Solid Edge part; units mm, degrees
sketch "Sketch1" plane through (0, 0, 0) normal (0, -1, 0) x (1, 0, 0)
  line L0 (0, 0) -> (9, 0)
  line L1 (9, 0) -> (7.5, 3)
  line L2 (7.5, 3) -> (0, 3)
  dimension "D1" = 9
  dimension "D2" = 7.5
revolve "RevolvedProtrusion1" add sketch "Sketch1" angle 360 about axis through (0, 0, 3) along (0, 0, -1)
sketch "Sketch2" plane through (0, 0, 3) normal (0, 0, 1) x (1, 0, 0)
  line L0 (0, 4.6188) -> (-4, -2.3094)
  line L1 (-4, -2.3094) -> (4, -2.3094)
  line L2 (4, -2.3094) -> (0, 4.6188)
  dimension "D1" = 4
extrude "triangle_cut" cut sketch "Sketch2" against normal blind 0.5
fillet "Round1" radius 0.25 5 edges at (-9, 0, 0) (-7.5, 0, 3) (-2, 1.1547, 3) (2, 1.1547, 3) (0, -2.3094, 3)
properties material "Polyethylene, low density"
Here's how the part is built. I have some questions about the finished solid (model axes, mm). A direction names the side the tool comes from. Coordinates: 2 decimals unless noted, no trailing zeros. Order: outer loops, then holes, each group sorted by start corner. A loop starts at its lowest first (then second) coordinate and runs counter-clockwise, first axis right, second up. Notation, with made-up numbers: M -33.5,89 L 24.5,89 A22 ccw 24.5,105 Z; hole C 81,-1.5 d3. An arc over 180 degrees is marked long. Answer as a JSON object with one key per item and string values. Group by question number.
(1) Which directions (+Z, -Z, +X, -X, +Y, -Y) give clear straight access to the entire face, cutting with the end or side of a thin tool? Please do faces 5 (the face through (2.03, 1.24, 2.92)), 6 (the face through (0, 0, 0)).
(2) Suppose I cut it at A-A, the plane z = 1.95. Please give me the cut outline in (x, y) (3 decimals), then the cut area to 3 significant figures.
(3) If we mould it in two halves opening along Y, with no side actions, what happens to faces 1 (the face through (3.2, -0.1, 3)), 2 (the face through (-2.093, 1.137, 2.925)), 3 (the face through (0, 0, 2.5)), 4 (the face through (7.29, -2.3, 2.71))? For each: released by +Y, released by -Y, zero draft, split by the parting line, or undercut.
(4) Suppose I cut it at B-B, the plane z = 0.85. Please give me the cut outline in (x, y) (3 decimals), then the cut area to 3 significant figures.
(5) I need wall thicknesses on probe 1 along Y at (x, z) = (1.75, 2.55); probe 2 along X at (y, z) = (-2.25, 2.65); probe 3 along X at (y, z) = (0, 0.4). Which ranges of each line are inside material? Lowest first, please.
Values found:
{
 "1": {"face 5": "+Z", "face 6": "-Z, +X, -X, +Y, -Y"},
 "2": {"outline": "C 0,0 d16.05", "area": "202 mm^2"},
 "3": {"face 1": "zero draft", "face 2": "undercut", "face 3": "undercut", "face 4": "split by the parting line"},
 "4": {"outline": "C 0,0 d17.15", "area": "231 mm^2"},
 "5": {"probe 1": "y = -7.52 to -2.31, 1.59 to 7.52", "probe 2": "x = -7.34 to -3.97, 3.97 to 7.34", "probe 3": "x = -8.8 to 8.8"}
}
